```python
from build123d import *
from build123d.topology import SkipClean

# Parameters (mm, degrees)
SKETCH1_W                      = 10
SKETCH1_H                      = 30
BOSS_EXTRUDE1_DEPTH            = 5.5
SKETCH2_R                      = 4.205
CUT_EXTRUDE1_DEPTH             = 19.848077
BOSS_EXTRUDE2_START            = -10
BOSS_EXTRUDE2_DEPTH            = 15
CUT_EXTRUDE_THIN1_DEPTH        = 24.683484
CUT_EXTRUDE_THIN1_DEPTH_BACK   = 1.5
CUT_EXTRUDE_THIN2_DEPTH        = 24.683484
CUT_EXTRUDE_THIN2_DEPTH_BACK   = 1.5
CBORE_FOR_M4_SHCS1_D           = 4.5
CBORE_FOR_M4_SHCS1_CBORE_D     = 8
CBORE_FOR_M4_SHCS1_CBORE_DEPTH = 4
SKETCH22_R                     = 4
CUT_EXTRUDE2_DEPTH             = 1.03126


with BuildPart() as part:
    # Sketch1 → Boss-Extrude1 (new body)
    with BuildSketch(Plane.XY):
        Rectangle(SKETCH1_W, SKETCH1_H)
    extrude(amount=BOSS_EXTRUDE1_DEPTH)

    # Sketch2 → Cut-Extrude1 (cut, through all)
    with BuildSketch(Plane(origin=(5, 0, 0), x_dir=(0, 0, -1), z_dir=(1, 0, 0))):
        with Locations((0.25, 0)):
            Circle(SKETCH2_R)
    extrude(amount=-CUT_EXTRUDE1_DEPTH, mode=Mode.SUBTRACT)

    # Sketch9 → Boss-Extrude2 (add)
    with SkipClean():  # the faces are left unmerged after this step: merging them gives an invalid solid
        with BuildSketch(Plane(origin=(5, 0, 0), x_dir=(0, 0, -1), z_dir=(1, 0, 0)).offset(BOSS_EXTRUDE2_START)):
            with BuildLine():
                ThreePointArc((-5.5, -9.119927), (-2.862491, -10.322207), (0, -10.778361))
                Line((0, -10.778361), (0, -4.197562))
                ThreePointArc((0, -4.197562), (-3.955, 0), (0, 4.197562))
                Line((0, 4.197562), (0, 10.778361))
                ThreePointArc((0, 10.778361), (-2.862491, 10.322207), (-5.5, 9.119927))
                Line((-5.5, 9.119927), (-5.5, -9.119927))
            make_face()
            with BuildLine():
                ThreePointArc((-5.5, 9.119927), (-10.53126, 0), (-5.5, -9.119927))
                Line((-5.5, -9.119927), (-5.5, 9.119927))
            make_face()
        extrude(amount=BOSS_EXTRUDE2_DEPTH)

    # Sketch12 → Cut-Extrude-Thin1 (cut, two sides: drawn at the far end of the back side and taken through both)
    with SkipClean():  # the faces are left unmerged after this step: merging them gives an invalid solid
        with BuildSketch(Plane(origin=(10, 0, 0), x_dir=(0, 0, -1), z_dir=(1, 0, 0)).offset(-CUT_EXTRUDE_THIN1_DEPTH_BACK)):
            Polygon((-0.125, 0.649519), (-9.461845, -4.741111), (-8.711845, -6.040149), (0.625, -0.649519), align=None)
        extrude(amount=CUT_EXTRUDE_THIN1_DEPTH + CUT_EXTRUDE_THIN1_DEPTH_BACK, mode=Mode.SUBTRACT)

    # Sketch21 → Cut-Extrude-Thin2 (cut, two sides: drawn at the far end of the back side and taken through both)
    with SkipClean():  # the faces are left unmerged after this step: merging them gives an invalid solid
        with BuildSketch(Plane(origin=(10, 0, 0), x_dir=(0, 0, -1), z_dir=(1, 0, 0)).offset(-CUT_EXTRUDE_THIN2_DEPTH_BACK)):
            Polygon((0.625, 0.649519), (-8.711845, 6.040149), (-9.461845, 4.741111), (-0.125, -0.649519), align=None)
        extrude(amount=CUT_EXTRUDE_THIN2_DEPTH + CUT_EXTRUDE_THIN2_DEPTH_BACK, mode=Mode.SUBTRACT)

    # CBORE for M4 SHCS1 (through all)
    with Locations(Plane.XY.offset(10.53126)):
        with Locations((0, 10), (0, -10)):
            CounterBoreHole(CBORE_FOR_M4_SHCS1_D / 2, CBORE_FOR_M4_SHCS1_CBORE_D / 2, CBORE_FOR_M4_SHCS1_CBORE_DEPTH)

    # Sketch22 → Cut-Extrude2 (cut)
    with SkipClean():  # the faces are left unmerged after this step: merging them gives an invalid solid
        with BuildSketch(Plane.XY.offset(6.53126)):
            with Locations((0, 10)):
                Circle(SKETCH22_R)
            with Locations((0, -10)):
                Circle(SKETCH22_R)
        extrude(amount=-CUT_EXTRUDE2_DEPTH, mode=Mode.SUBTRACT)


solid = part.part
```
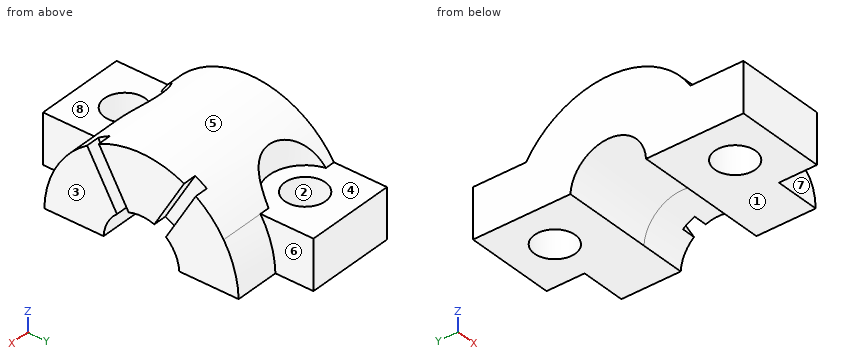
The listing builds one solid part. Answer for the finished solid, in the listing's coordinates (mm). Face numbers are marked on the shaded views. A direction names the side the tool comes from. Give positions to 0.01 mm unless a question says otherwise; leave off trailing zeros. Order: outer loops, then holes, each group sorted by start corner. A loop starts at its lowest first (then second) coordinate and runs counter-clockwise, first axis right, second up. Notation, with made-up numbers: (42, 0.5) -> (89, 0.5) arc R25 ccw to (89, 15.5) -> close; hole circle Ø2 at (22.25, 15). An arc over 180 degrees is marked (long way). Answer as a JSON object with one key per item and string values. Group by question number.
Item 1: A tool of negligible diameter and unlimited length cuts with its end or side. For the marked faces 4, 5, 6, 7 and 8, from which of +Z, -Z, +X, -X, +Y, -Y can it reach the whole face along a straight path? Write none if from no direction.
Item 2: The part is cut by section C-C on x = 4.25. Write down the section's boundary in (y, z) (3 decimals), and give its area (3 significant figures).
Item 3: Consider L1, parallel to Y at x = 0, z = 4; L2, parallel to X at y = 10, z = 3; L3, parallel to Y at x = 1.75, z = 4.25. Determine where each line is inside the solid, lowest interval first. Write a range as from..to.
Item 4: The part is cut by section A-A on x = 0. Write down the section's boundary in (y, z) (3 decimals).
Item 5: The part is cut by section B-B on y = -10. Write down the section's boundary in (x, z), and give its area (3 significant figures).
Item 6: Flat-ended cylindrical pins translate along their axes: pin 1 (2.5 mm diameter, centred on x = -1.5, y = -9.5, fed in from +Z); pin 2 (1.6 mm diameter, centred on y = -12, z = 3, fed in from +X); pin 3 (1 mm diameter, centred on x = 3.5, z = 7, fed in from -Y). Find the tip coordinate at first contact, or state that the pin passes through.
Item 7: The part is cut by section D-D on z = 9. Write down the section's boundary in (x, y).
Item 8: Determine the mould class of the marked faces 1, 2 and 3 for opening direction X: pulls with the +X half, pulls with the -X half, needs draft (parallel to the pull), parting line crosses it, or undercut.
Result set:
{
 "1": {"face 4": "+Z, +Y", "face 5": "+Z, +X, -X", "face 6": "+Z, +X, +Y", "face 7": "+Z, +X, -Y", "face 8": "+Z, -Y"},
 "2": {"outline": "(-15, 0) -> (-4.198, 0) arc R4.205 cw to (4.198, 0) -> (15, 0) -> (15, 5.5) -> (9.12, 5.5) arc R10.781 ccw to (-9.12, 5.5) -> (-15, 5.5) -> close", "area": "204 mm²"},
 "3": {"L1": "-15..-12.25, -7.75..7.75, 12.25..15", "L2": "-5..-2.25, 2.25..10", "L3": "-15..-11.41, -8.59..8.59, 11.41..15"},
 "4": {"outline": "(-15, 0) -> (-12.25, 0) -> (-12.25, 5.5) -> (-15, 5.5) -> close; (-7.75, 0) -> (-4.198, 0) arc R4.205 cw to (4.198, 0) -> (7.75, 0) -> (7.75, 5.5) -> (6, 5.5) -> (6, 8.707) arc R10.781 ccw to (-6, 8.707) -> (-6, 5.5) -> (-7.75, 5.5) -> close; (12.25, 0) -> (15, 0) -> (15, 5.5) -> (12.25, 5.5) -> close"},
 "5": {"outline": "(-5, 0) -> (-2.25, 0) -> (-2.25, 5.5) -> (-5, 5.5) -> close; (2.25, 0) -> (10, 0) -> (10, 3.78) -> (5, 3.78) -> (5, 5.5) -> (2.25, 5.5) -> close", "area": "49.1 mm²"},
 "6": {"pin 1": "z = 5.5", "pin 2": "x = 5", "pin 3": "y = -8.39"},
 "7": {"outline": "(-5, -5.54) -> (8.5, -5.54) -> (8.5, -4.47) -> (10, -4.47) -> (10, 4.47) -> (8.5, 4.47) -> (8.5, 5.54) -> (-5, 5.54) -> close"},
 "8": {"face 1": "needs draft", "face 2": "undercut", "face 3": "pulls with the +X half"}
}
